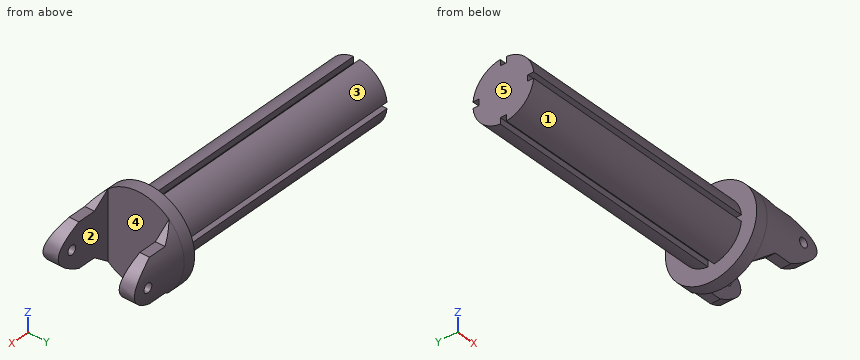
```python
from build123d import *

# Parameters (mm, degrees)
BOSS_EXTRUDE1_DEPTH     = 40
SKETCH2_R               = 7.5
BOSS_EXTRUDE2_DEPTH     = 2
BOSS_EXTRUDE3_DEPTH     = 10
CUT_EXTRUDE1_DEPTH      = 55.004629431
CUT_EXTRUDE1_DEPTH_BACK = 55.004629431
CUT_EXTRUDE2_DEPTH      = 54.619586107
CUT_EXTRUDE2_DEPTH_BACK = 54.619586107
SKETCH5_R               = 0.75


with BuildPart() as part:
    # Sketch1 → Boss-Extrude1 (new body)
    with BuildSketch(Plane(origin=(0, 0, 0), x_dir=(0, 0, -1), z_dir=(1, 0, 0))):
        with BuildLine():
            Line((-0.5, 4), (0.5, 4))
            Line((0.5, 4), (0.5, 4.974937186))
            ThreePointArc((0.5, 4.974937186), (3.535533906, 3.535533906), (4.974937186, 0.5))
            Line((4.974937186, 0.5), (4, 0.5))
            Line((4, 0.5), (4, -0.5))
            Line((4, -0.5), (4.974937186, -0.5))
            ThreePointArc((4.974937186, -0.5), (3.535533906, -3.535533906), (0.5, -4.974937186))
            Line((0.5, -4.974937186), (0.5, -4))
            Line((0.5, -4), (-0.5, -4))
            Line((-0.5, -4), (-0.5, -4.974937186))
            ThreePointArc((-0.5, -4.974937186), (-3.535533906, -3.535533906), (-4.974937186, -0.5))
            Line((-4.974937186, -0.5), (-4, -0.5))
            Line((-4, -0.5), (-4, 0.5))
            Line((-4, 0.5), (-4.974937186, 0.5))
            ThreePointArc((-4.974937186, 0.5), (-3.535533906, 3.535533906), (-0.5, 4.974937186))
            Line((-0.5, 4.974937186), (-0.5, 4))
        make_face()
    extrude(amount=BOSS_EXTRUDE1_DEPTH)

    # Sketch2 → Boss-Extrude2 (add)
    with BuildSketch(Plane(origin=(40, 0, 0), x_dir=(0, 0, -1), z_dir=(1, 0, 0))):
        Circle(SKETCH2_R)
    extrude(amount=BOSS_EXTRUDE2_DEPTH)

    # Sketch3 → Boss-Extrude3 (add)
    with BuildSketch(Plane(origin=(42, 0, 0), x_dir=(0, 0, -1), z_dir=(1, 0, 0))):
        with BuildLine():
            ThreePointArc((5.590169944, 5), (0, 7.5), (-5.590169944, 5))
            Line((-5.590169944, 5), (-4.898979486, 5))
            Line((-4.898979486, 5), (4.898979486, 5))
            Line((4.898979486, 5), (5.590169944, 5))
        make_face()
        with BuildLine():
            Line((-4.898979486, -5), (-5.590169944, -5))
            ThreePointArc((-5.590169944, -5), (0, -7.5), (5.590169944, -5))
            Line((5.590169944, -5), (4.898979486, -5))
            Line((4.898979486, -5), (-4.898979486, -5))
        make_face()
    extrude(amount=BOSS_EXTRUDE3_DEPTH)

    # Sketch4 → Cut-Extrude1 (cut, two sides: drawn at the far end of the back side and taken through both)
    with BuildSketch(Plane.XZ.offset(-5).offset(-CUT_EXTRUDE1_DEPTH_BACK)):
        with BuildLine():
            Line((42, 5.590169944), (52, 5.590169944))
            Line((52, 5.590169944), (52, -5.590169944))
            Line((52, -5.590169944), (42, -5.590169944))
            Line((42, -5.590169944), (44.640400827, -3.590169944))
            Line((44.640400827, -3.590169944), (47.640400827, -3.590169944))
            add(Edge.make_bspline(
                [(47.640400827, -3.590169944), (50.280133609, -2.393446629), (52.919866391, 0), (50.280133609, 2.393446629), (47.640400827, 3.590169944)],
                knots=[0.178885438, 0.178885438, 0.178885438, 0.178885438, 0.5, 0.821114562, 0.821114562, 0.821114562, 0.821114562], degree=3))
            Line((47.640400827, 3.590169944), (44.640400827, 3.590169944))
            Line((44.640400827, 3.590169944), (42, 5.590169944))
        make_face()
    extrude(amount=CUT_EXTRUDE1_DEPTH + CUT_EXTRUDE1_DEPTH_BACK, mode=Mode.SUBTRACT)

    # Sketch5 → Cut-Extrude2 (cut, two sides: drawn at the far end of the back side and taken through both)
    with BuildSketch(Plane.XZ.offset(-5).offset(-CUT_EXTRUDE2_DEPTH_BACK)):
        with Locations(Location((49, 0, 0), (0, 0, 270))):
            Circle(SKETCH5_R)
    extrude(amount=CUT_EXTRUDE2_DEPTH + CUT_EXTRUDE2_DEPTH_BACK, mode=Mode.SUBTRACT)


solid = part.part
```
Could you check a few things on this model? Use its own coordinates, in mm. Face numbers are marked on the shaded views. A direction names the side the tool comes from. Round coordinates to 2 decimals unless told otherwise and drop trailing zeros. Order: outer loops, then holes, each group sorted by start corner. A loop starts at its lowest first (then second) coordinate and runs counter-clockwise, first axis right, second up. Notation, with made-up numbers: (85.5, 26) -> (103.5, 26) arc R22 ccw to (103.5, 54) -> close; hole circle Ø8 at (86, 34). An arc over 180 degrees is marked (long way). One line per question, with ' | ' between items.
Q1. If I drill on line 1 (X direction, y = 5.85, z = 0); line 2 (Y direction, x = 47.5, z = 0.25); line 3 (X direction, y = 0.75, z = 6.5), over which ranges is the centre line in solid material (lowest first)? Write a range as from..to.
Computed values:
line 1: 40..48.25, 49.75..51.6 | line 2: -7.5..-5, 5..7.5 | line 3: 40..42
Q2. We'd pull the mould along Y, two halves only. Please class the marked faces 3, 4 and 5: released by +Y, released by -Y, zero draft, split by the parting line, or undercut.
Computed values:
face 3: released by +Y | face 4: undercut | face 5: zero draft
Q3. Which directions (+Z, -Z, +X, -X, +Y, -Y) give clear straight access to the entire face, cutting with the end or side of a thin tool? Please do the marked faces 1 and 2.
Computed values:
face 1: -Z, -X, -Y | face 2: +Z, -Z, +X
Q4. If we section it at B-B on z = 0: Give the number of separate pieces and of enclosed holes in the cut face, plus the area to 4 significant figures.
Computed values:
separate pieces: 3 | enclosed holes: 0 | area: 390.5 mm²
Q5. If we section it at C-C on y = 0: Write out the boundary of the cut face in (x, z), plus the area to 3 significant figures.
Computed values:
outline: (0, -4) -> (40, -4) -> (40, -7.5) -> (42, -7.5) -> (42, 7.5) -> (40, 7.5) -> (40, 4) -> (0, 4) -> close | area: 350 mm²
Q6. I'm going to push flat-ended pins straight in: pin 1 (1.1 mm diameter, centred on x = 21, y = -4.5, fed in from +Z); pin 2 (1.1 mm diameter, centred on x = 21, y = -4.5, fed in from -Z); pin 3 (5 mm diameter, centred on x = 45, z = -1, fed in from +Y); pin 4 (1.5 mm diameter, centred on y = -3.5, z = -3.5, fed in from +X). Where does each tip first touch, or does it pass through?
Computed values:
pin 1: z = 3.07 | pin 2: z = -3.07 | pin 3: y = 7.5 | pin 4: x = 42
Q7. If we section it at A-A on x = 4.5: Write out the boundary of the cut face in (y, z), plus the area to 3 significant figures.
Computed values:
outline: (-4.97, -0.5) arc R5 ccw to (-0.5, -4.97) -> (-0.5, -4) -> (0.5, -4) -> (0.5, -4.97) arc R5 ccw to (4.97, -0.5) -> (4, -0.5) -> (4, 0.5) -> (4.97, 0.5) arc R5 ccw to (0.5, 4.97) -> (0.5, 4) -> (-0.5, 4) -> (-0.5, 4.97) arc R5 ccw to (-4.97, 0.5) -> (-4, 0.5) -> (-4, -0.5) -> close | area: 74.6 mm²
